```python
from build123d import *

# Parameters (mm, degrees)
SKETCH1_W           = 280
SKETCH1_H           = 70
BOSS_EXTRUDE1_DEPTH = 30
SKETCH2_R           = 5.5
CUT_EXTRUDE1_DEPTH  = 80


with BuildPart() as part:
    # Sketch1 → Boss-Extrude1 (new body)
    with BuildSketch(Plane.XY):
        Rectangle(SKETCH1_W, SKETCH1_H)
    extrude(amount=BOSS_EXTRUDE1_DEPTH)

    # Sketch2 → Cut-Extrude1 (cut)
    with BuildSketch(Plane(origin=(0, 35, 0), x_dir=(1, 0, 0), z_dir=(0, 1, 0))):
        with Locations(Location((-65, -15, 0), (0, 0, 270))):
            Circle(SKETCH2_R)
        with Locations(Location((65, -15, 0), (0, 0, 270))):
            Circle(SKETCH2_R)
    extrude(amount=-CUT_EXTRUDE1_DEPTH, mode=Mode.SUBTRACT)


solid = part.part
```
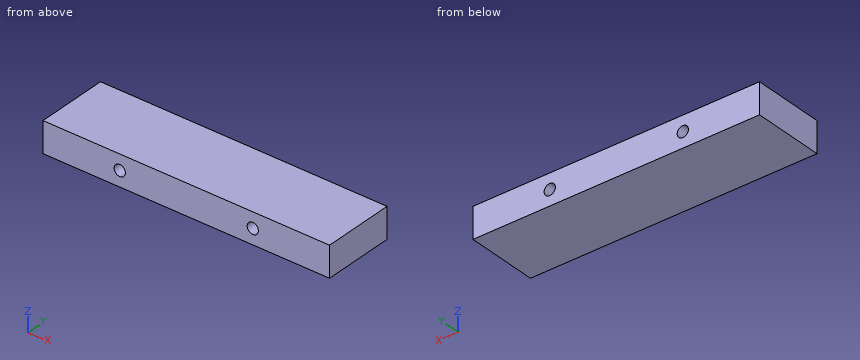
Verification items for the finished model (mm, model axes). Round coordinates to 2 decimals unless told otherwise and drop trailing zeros. Write each loop counter-clockwise with the first axis right and the second up, starting at its lowest first coordinate (ties: lowest second). Pieces come first, ordered by that corner, then holes. Notation, with made-up numbers: (13, 75.25) - (62, 75.25) arc R25 cw to (62, 91.25) - close; hole circle Ø9 at (50.25, 28.25). An arc over 180 degrees is marked (long way). Answer as a JSON object with one key per item and string values. Group by question number.
Q1. Thickness scan on line 1 (X direction, y = 10, z = 15); line 2 (X direction, y = 7, z = 16.75). Record the ranges inside material, lowest first.
Q2. Section check C-C, the plane y = -26. Enter the section's corners in (x, z).
Q3. Section check A-A, the plane x = -65. Enter the section's corners in (y, z).
Q4. Go/stop test with a flat-tipped pin: pin 1 Ø10 at (x, z) = (65, 15) entering from +Y. Record where the tip stops, or that it passes through.
Q5. Section check B-B, the plane z = 15. Enter the section's corners in (x, y), plus the area to 3 significant figures.
Found:
{
 "1": {"line 1": "x = -140 to -70.5, -59.5 to 59.5, 70.5 to 140", "line 2": "x = -140 to -70.21, -59.79 to 59.79, 70.21 to 140"},
 "2": {"outline": "(-140, 0) - (140, 0) - (140, 30) - (-140, 30) - close; hole circle Ø11 at (-65, 15); hole circle Ø11 at (65, 15)"},
 "3": {"outline": "(-35, 0) - (35, 0) - (35, 9.5) - (-35, 9.5) - close; (-35, 20.5) - (35, 20.5) - (35, 30) - (-35, 30) - close"},
 "4": {"pin 1": "passes through"},
 "5": {"outline": "(-140, -35) - (-70.5, -35) - (-70.5, 35) - (-140, 35) - close; (-59.5, -35) - (59.5, -35) - (59.5, 35) - (-59.5, 35) - close; (70.5, -35) - (140, -35) - (140, 35) - (70.5, 35) - close", "area": "18,100 mm^2"}
}
